Could you check a few things on this model? Use its own coordinates, in mm. A direction names the side the tool comes from. Give positions to 0.01 mm unless a question says otherwise; leave off trailing zeros. Loops run counter-clockwise (first coordinate to the right, second up) from the corner with the lowest first, then second, coordinate; pieces in that order, holes last. Notation, with made-up numbers: (-19, 44.25) -> (39, 44.25) arc R22 ccw to (39, 55.25) -> close; hole circle Ø6 at (7, -32). An arc over 180 degrees is marked (long way). Put each result on its own line as item: value.
```python
from build123d import *

# Parameters (mm, degrees)
SKETCH1_W           = 90
SKETCH1_H           = 60
BOSS_EXTRUDE1_DEPTH = 4
SKETCH2_R           = 2.15
SKETCH2_R_2         = 1.7
CUT_EXTRUDE1_DEPTH  = 4
CUT_EXTRUDE2_DEPTH  = 2
CUT_EXTRUDE3_DEPTH  = 2
FILLET3_R           = 5


with BuildPart() as part:
    # Sketch1 → Boss-Extrude1 (new body)
    with BuildSketch(Plane(origin=(0, 0, 0), x_dir=(1, 0, 0), z_dir=(0, 1, 0))):
        Rectangle(SKETCH1_W, SKETCH1_H)
    extrude(amount=BOSS_EXTRUDE1_DEPTH)

    # Sketch2 → Cut-Extrude1 (cut)
    with BuildSketch(Plane(origin=(0, 4, 0), x_dir=(1, 0, 0), z_dir=(0, 1, 0))):
        with Locations(Location((-34.3999999, -0.00262532, 0), (0, 0, 270))):
            Circle(SKETCH2_R)
        with Locations(Location((34.400000034, 0.00039051, 0), (0, 0, 270))):
            Circle(SKETCH2_R)
        with Locations(Location((-39, 24, 0), (0, 0, 270))):
            Circle(SKETCH2_R_2)
        with Locations(Location((-39, -24, 0), (0, 0, 270))):
            Circle(SKETCH2_R_2)
        with Locations(Location((39, -24, 0), (0, 0, 270))):
            Circle(SKETCH2_R_2)
        with Locations(Location((39, 24, 0), (0, 0, 270))):
            Circle(SKETCH2_R_2)
    extrude(amount=-CUT_EXTRUDE1_DEPTH, mode=Mode.SUBTRACT)

    # Sketch3 → Cut-Extrude2 (cut)
    with BuildSketch(Plane(origin=(0, 4, 0), x_dir=(1, 0, 0), z_dir=(0, 1, 0))):
        Polygon((-30.8249999, 2.061401893), (-34.3999999, 4.125429105), (-37.9749999, 2.061401893), (-37.9749999, -2.066652532), (-34.3999999, -4.130679744), (-30.8249999, -2.066652532), align=None)
        Polygon((37.975000034, 2.064417722), (34.400000034, 4.128444934), (30.825000034, 2.064417722), (30.825000034, -2.063636703), (34.400000034, -4.127663915), (37.975000034, -2.063636703), align=None)
    extrude(amount=-CUT_EXTRUDE2_DEPTH, mode=Mode.SUBTRACT)

    # Sketch4 → Cut-Extrude3 (cut)
    with BuildSketch(Plane.XZ):
        Polygon((-36.2, 25.616580754), (-39, 27.233161507), (-41.8, 25.616580754), (-41.8, 22.383419246), (-39, 20.766838493), (-36.2, 22.383419246), align=None)
        Polygon((-36.2, -22.383419246), (-39, -20.766838493), (-41.8, -22.383419246), (-41.8, -25.616580754), (-39, -27.233161507), (-36.2, -25.616580754), align=None)
        Polygon((41.8, -22.383419246), (39, -20.766838493), (36.2, -22.383419246), (36.2, -25.616580754), (39, -27.233161507), (41.8, -25.616580754), align=None)
        Polygon((41.8, 25.616580754), (39, 27.233161507), (36.2, 25.616580754), (36.2, 22.383419246), (39, 20.766838493), (41.8, 22.383419246), align=None)
    extrude(amount=-CUT_EXTRUDE3_DEPTH, mode=Mode.SUBTRACT)

    # Fillet3
    fillet3_edges = [part.edges().sort_by_distance(p)[0] for p in [
        (-45, 2, -30),
        (45, 2, -30),
        (45, 2, 30),
        (-45, 2, 30),
    ]]
    fillet(fillet3_edges, radius=FILLET3_R)


solid = part.part
```
1. For faces 4 (the face through (-40.42, 0.986, 21.586)), 5 (the face through (30.825, 3, 0)), 6 (the face through (-45, 2, 0)), which set-ups out of +Z, -Z, +X, -X, +Y, -Y let a thin tool reach every point of the face, with its end or its side?
Recorded:
face 4: -Y
face 5: +Y
face 6: +Z, -Z, -X, +Y, -Y
2. I'm going to push flat-ended pins straight in: pin 1 (3 mm diameter, centred on x = -38.5, z = -22.5, fed in from -Y); pin 2 (5.5 mm diameter, centred on x = 39, z = -24, fed in from -Y). Where does each tip first touch, or does it pass through?
Recorded:
pin 1: stops at y = 0
pin 2: stops at y = 2
3. I need wall thicknesses on line 1 (X direction, y = 2.4, z = 24); line 2 (X direction, y = 2.4, z = 1) (3 decimals); line 3 (Y direction, x = -35, z = 2.5). Which ranges of each line are inside material? Lowest first, please.
Recorded:
line 1: x = -45 to -40.7, -37.3 to 37.3, 40.7 to 45
line 2: x = -45 to -37.975, -30.825 to 30.825, 37.975 to 45
line 3: y = 0 to 2
4. If we section it at A-A (z = 0): List the corners of the cut face in (x, y) for me (3 decimals), then the cut area to 3 significant figures.
Recorded:
outline: (-45, 0) -> (-36.55, 0) -> (-36.55, 2) -> (-37.975, 2) -> (-37.975, 4) -> (-45, 4) -> close; (-32.25, 0) -> (32.25, 0) -> (32.25, 2) -> (30.825, 2) -> (30.825, 4) -> (-30.825, 4) -> (-30.825, 2) -> (-32.25, 2) -> close; (36.55, 0) -> (45, 0) -> (45, 4) -> (37.975, 4) -> (37.975, 2) -> (36.55, 2) -> close
area: 314 mm^2
5. Thinking about a two-plate mould opening in X: for faces 1 (the face through (43, 2, 29)), 2 (the face through (-44, 2, -28)), 3 (the face through (-40.42, 0.986, -26.414)), which applies, pulls with the +X half, pulls with the -X half, needs draft (parallel to the pull), parting line crosses it, or undercut?
Recorded:
face 1: pulls with the +X half
face 2: pulls with the -X half
face 3: undercut
6. If we section it at B-B (z = -24): List the corners of the cut face in (x, y) for me, then the cut area to 3 significant figures.
Recorded:
outline: (-45, 0) -> (-41.8, 0) -> (-41.8, 2) -> (-40.7, 2) -> (-40.7, 4) -> (-45, 4) -> close; (-37.3, 2) -> (-36.2, 2) -> (-36.2, 0) -> (36.2, 0) -> (36.2, 2) -> (37.3, 2) -> (37.3, 4) -> (-37.3, 4) -> close; (40.7, 2) -> (41.8, 2) -> (41.8, 0) -> (45, 0) -> (45, 4) -> (40.7, 4) -> close
area: 324 mm^2
